```python
from build123d import *

# Parameters (mm, degrees)
SKETCH1_W          = 623.55984
SKETCH1_H          = 78.16342
BASE_FLANGE1_DEPTH = 1.5875
SKETCH3_R          = 2.75
SKETCH3_R_2        = 2.921
SKETCH3_W          = 32.08
SKETCH3_H          = 32.08
CUT_EXTRUDE3_DEPTH = 389.990867909


# Sheet-metal steps are written as plain solids
with BuildPart() as part:
    # Sketch1 → Base-Flange1 (new body)
    with BuildSketch(Plane.XY):
        with Locations((-38.857061865, -129.337653818)):
            Rectangle(SKETCH1_W, SKETCH1_H)
    extrude(amount=-BASE_FLANGE1_DEPTH)

    # Sketch3 → Cut-Extrude3 (cut, through all)
    with BuildSketch(Plane.XY):
        with Locations((92.914515529, -110.369060902)):
            Circle(SKETCH3_R)
        with Locations((35.391947046, -147.147547142)):
            Circle(SKETCH3_R_2)
        with Locations((-172.247688202, -111.060995593)):
            Circle(SKETCH3_R_2)
        with Locations((-223.059163384, -156.664689794)):
            Circle(SKETCH3_R_2)
        with Locations((-304.149901865, -121.952427932)):
            Rectangle(SKETCH3_W, SKETCH3_H)
        with Locations((-86.931641865, -121.952427932)):
            Rectangle(SKETCH3_W, SKETCH3_H)
        with Locations((12.392518135, -121.952427932)):
            Rectangle(SKETCH3_W, SKETCH3_H)
        with Locations((229.610778135, -121.952427932)):
            Rectangle(SKETCH3_W, SKETCH3_H)
    extrude(amount=-CUT_EXTRUDE3_DEPTH, mode=Mode.SUBTRACT)


solid = part.part
```
Can you work these out from the model? Positions are in its coordinate system, mm. Give positions to 0.01 mm unless a question says otherwise; leave off trailing zeros. Loops run counter-clockwise (first coordinate to the right, second up) from the corner with the lowest first, then second, coordinate; pieces in that order, holes last. Notation, with made-up numbers: M -36,39 L -4,39 A16 ccw -4,48 Z; hole C 48,59.5 d4. An arc over 180 degrees is marked long. Use CSV: the item, a comma, the result in double quotes. Start each with the question number.
1. Imagine slicing it at C-C, the plane z = -1.2. Count the separate pieces of the cut face and the enclosed holes in it, plus the area to 3 significant figures.
2. Imagine slicing it at B-B, the plane x = -78. Write out the boundary of the cut face in (y, z).
3. For P1, Ø4.5, axis at x = 92.91, y = -110.37, coming from the +Z side, with a flat end and sliding along its axis, tell me the tip position at first contact or that it passes through.
4. Imagine slicing it at A-A, the plane y = -130. Write out the boundary of the cut face in (x, z), plus the area to 3 significant figures.
5. If I drill on L1, parallel to X at y = -137, z = -0.35; L2, parallel to Y at x = 20, z = -1.5; L3, parallel to X at y = -155, z = -0.6, over which ranges is the centre line in solid material (lowest first)?
Response values:
1,separate pieces,"1"
1,enclosed holes,"8"
1,area,"44,500 mm^2"
2,outline,"M -168.42,-1.59 L -137.99,-1.59 L -137.99,0 L -168.42,0 Z; M -105.91,-1.59 L -90.26,-1.59 L -90.26,0 L -105.91,0 Z"
3,P1,"through"
4,outline,"M -350.64,-1.59 L -320.19,-1.59 L -320.19,0 L -350.64,0 Z; M -288.11,-1.59 L -102.97,-1.59 L -102.97,0 L -288.11,0 Z; M -70.89,-1.59 L -3.65,-1.59 L -3.65,0 L -70.89,0 Z; M 28.43,-1.59 L 213.57,-1.59 L 213.57,0 L 28.43,0 Z; M 245.65,-1.59 L 272.92,-1.59 L 272.92,0 L 245.65,0 Z"
4,area,"786 mm^2"
5,L1,"-350.64 to -320.19, -288.11 to -102.97, -70.89 to -3.65, 28.43 to 213.57, 245.65 to 272.92"
5,L2,"-168.42 to -137.99, -105.91 to -90.26"
5,L3,"-350.64 to -225.46, -220.66 to 272.92"
